```python
from build123d import *

# Parameters (mm, degrees)
SKETCH1_W           = 42
SKETCH1_H           = 10
SKETCH1_R           = 2.45
SKETCH1_R_2         = 2.5
SKETCH1_R_3         = 2.55
SKETCH1_R_4         = 2.6
SKETCH1_R_5         = 2.65
BOSS_EXTRUDE1_DEPTH = 7
FILLET2_R           = 3


with BuildPart() as part:
    # Sketch1 → Boss-Extrude1 (new body)
    with BuildSketch(Plane(origin=(0, 0, 0), x_dir=(1, 0, 0), z_dir=(0, 1, 0))):
        with Locations((16, 0)):
            Rectangle(SKETCH1_W, SKETCH1_H)
        Circle(SKETCH1_R, mode=Mode.SUBTRACT)
        with Locations((8, 0)):
            Circle(SKETCH1_R_2, mode=Mode.SUBTRACT)
        with Locations((16, 0)):
            Circle(SKETCH1_R_3, mode=Mode.SUBTRACT)
        with Locations((24, 0)):
            Circle(SKETCH1_R_4, mode=Mode.SUBTRACT)
        with Locations((32, 0)):
            Circle(SKETCH1_R_5, mode=Mode.SUBTRACT)
    extrude(amount=BOSS_EXTRUDE1_DEPTH)

    # Fillet2
    fillet2_edges = [part.edges().sort_by_distance(p)[0] for p in [
        (-5, 3.5, 5),
        (-5, 3.5, -5),
    ]]
    fillet(fillet2_edges, radius=FILLET2_R)


solid = part.part
```
Input: part model. Units: mm. Frame: model coordinates. Round coordinates to 2 decimals unless told otherwise and drop trailing zeros. Loops run counter-clockwise (first coordinate to the right, second up) from the corner with the lowest first, then second, coordinate; pieces in that order, holes last. Notation, with made-up numbers: (-29, -35) -> (3, -35) arc R20 cw to (3, -29) -> close; hole circle Ø7 at (-16.5, 10). An arc over 180 degrees is marked (long way). One line per item, written item: value.
(1) Section A-A (x = 0). Return the cut outline in (y, z).
Geometry check:
outline: (0, -5) -> (7, -5) -> (7, -2.45) -> (0, -2.45) -> close; (0, 2.45) -> (7, 2.45) -> (7, 5) -> (0, 5) -> close
(2) Material intervals for line 1 (X direction, y = 4.25, z = 0); line 2 (Z direction, x = 32, y = 3.75); line 3 (X direction, y = 4.25, z = -0.75), sorted ascending. Write a range as [from, to].
Geometry check:
line 1: [-5, -2.45], [2.45, 5.5], [10.5, 13.45], [18.55, 21.4], [26.6, 29.35], [34.65, 37]
line 2: [-5, -2.65], [2.65, 5]
line 3: [-5, -2.33], [2.33, 5.62], [10.38, 13.56], [18.44, 21.51], [26.49, 29.46], [34.54, 37]
(3) Section C-C (z = -1.5). Return the cut outline in (x, y).
Geometry check:
outline: (-5, 0) -> (-1.94, 0) -> (-1.94, 7) -> (-5, 7) -> close; (1.94, 0) -> (6, 0) -> (6, 7) -> (1.94, 7) -> close; (10, 0) -> (13.94, 0) -> (13.94, 7) -> (10, 7) -> close; (18.06, 0) -> (21.88, 0) -> (21.88, 7) -> (18.06, 7) -> close; (26.12, 0) -> (29.82, 0) -> (29.82, 7) -> (26.12, 7) -> close; (34.18, 0) -> (37, 0) -> (37, 7) -> (34.18, 7) -> close
(4) Mould query, pull axis Z, two halves, no side actions, for faces 1 (the face through (16, 0, -3)), 2 (the face through (-4.14, 3.55, -4.1)), 3 (the face through (-0.5, 3.5, 2.4)). Classes: pulls with the +Z half, pulls with the -Z half, needs draft (parallel to the pull), parting line crosses it, or undercut.
Geometry check:
face 1: needs draft
face 2: pulls with the -Z half
face 3: undercut
(5) Section B-B (y = 3.75). Return the cut outline in (x, z).
Geometry check:
outline: (-5, -2) arc R3 ccw to (-2, -5) -> (37, -5) -> (37, 5) -> (-2, 5) arc R3 ccw to (-5, 2) -> close; hole circle Ø4.9 at (0, 0); hole circle Ø5 at (8, 0); hole circle Ø5.1 at (16, 0); hole circle Ø5.2 at (24, 0); hole circle Ø5.3 at (32, 0)
(6) Section D-D (x = 24). Return the cut outline in (y, z).
Geometry check:
outline: (0, -5) -> (7, -5) -> (7, -2.6) -> (0, -2.6) -> close; (0, 2.6) -> (7, 2.6) -> (7, 5) -> (0, 5) -> close
